```python
from build123d import *

# Parameters (mm, degrees)
F0_R     = 9
F1_DEPTH = 3


with BuildPart() as f1:
    # F0 (on Front) → F1 (new body)
    with BuildSketch(Plane.XZ):
        with BuildLine():
            Line((1.35, 24.837218), (1.35, 13.856218))
            Line((1.35, 13.856218), (-1.35, 13.856218))
            Line((-1.35, 13.856218), (-1.35, 24.837218))
            ThreePointArc((-1.35, 24.837218), (-9.30431, 23.022838), (-16.250873, 18.744019))
            Line((-16.250873, 18.744019), (-8.48636, 10.979053))
            Line((-8.48636, 10.979053), (-10.424493, 9.099692))
            Line((-10.424493, 9.099692), (-18.189233, 16.864432))
            ThreePointArc((-18.189233, 16.864432), (-22.849106, 9.663922), (-24.801066, 1.312179))
            Line((-24.801066, 1.312179), (-13.820066, 1.312179))
            Line((-13.820066, 1.312179), (-13.811545, -1.388101))
            Line((-13.811545, -1.388101), (-24.792545, -1.388101))
            ThreePointArc((-24.792545, -1.388101), (-22.854652, -9.674423), (-18.233002, -16.819974))
            Line((-18.233002, -16.819974), (-10.468263, -9.055235))
            Line((-10.468263, -9.055235), (-8.311446, -11.123312))
            Line((-8.311446, -11.123312), (-16.075972, -18.887838))
            ThreePointArc((-16.075972, -18.887838), (-8.894515, -23.145882), (-0.707747, -24.78329))
            Line((-0.707747, -24.78329), (-0.69587, -13.802296))
            Line((-0.69587, -13.802296), (2.003764, -13.757801))
            Line((2.003764, -13.757801), (1.70544, -24.734748))
            ThreePointArc((1.70544, -24.734748), (9.667631, -22.834323), (16.579394, -18.44848))
            Line((16.579394, -18.44848), (8.911142, -10.588437))
            Line((8.911142, -10.588437), (10.82033, -8.679249))
            Line((10.82033, -8.679249), (18.48873, -16.539148))
            ThreePointArc((18.48873, -16.539148), (22.915536, -9.529923), (24.788649, -1.4542))
            Line((24.788649, -1.4542), (13.807649, -1.4542))
            Line((13.807649, -1.4542), (13.823381, 1.245754))
            Line((13.823381, 1.245754), (24.804381, 1.2458))
            ThreePointArc((24.804381, 1.2458), (22.970893, 9.47684), (18.488676, 16.619769))
            Line((18.488676, 16.619769), (10.723937, 8.85503))
            Line((10.723937, 8.85503), (8.814749, 10.764218))
            Line((8.814749, 10.764218), (16.579488, 18.528958))
            ThreePointArc((16.579488, 18.528958), (9.50343, 22.98359), (1.35, 24.837218))
        make_face()
        Circle(F0_R, mode=Mode.SUBTRACT)
    extrude(amount=F1_DEPTH)


solid = f1.part
```
Read the model definition and answer for the solid it produces. Units are mm, in the model's axes. A direction names the side the tool comes from. Coordinates: 2 decimals unless noted, no trailing zeros. Order: outer loops, then holes, each group sorted by start corner. A loop starts at its lowest first (then second) coordinate and runs counter-clockwise, first axis right, second up. Notation, with made-up numbers: (-29.75, 41.5) - (-3.75, 41.5) arc R25 cw to (-3.75, 66.5) - close; hole circle Ø5 at (34.25, -3). An arc over 180 degrees is marked (long way). Answer as a JSON object with one key per item and string values. Group by question number.
Item 1: Section A-A (x = 12.5) is taken. Give the vertices of the cut face in (y, z), plus the area to 3 significant figures.
Item 2: Section D-D (x = 0) is taken. Give the vertices of the cut face in (y, z), plus the area to 3 significant figures.
Item 3: Section C-C (z = 14.5) is taken. Give the vertices of the cut face in (x, y), plus the area to 3 significant figures.
Item 4: Flat-ended cylindrical pins translate along their axes: P1, Ø1.5, axis at y = -1, z = 18, coming from the +X side; P2, Ø1.5, axis at x = 20, y = -2, coming from the +Z side; P3, Ø0.9, axis at x = 21.5, y = -2, coming from the -Z side; P4, Ø11, axis at x = 0, z = 0, coming from the -Y side. Find the tip coordinate at first contact, or state that the pin passes through.
Item 5: Consider probe 1 along Z at (x, y) = (0, -1.05); probe 2 along Z at (x, y) = (12, -1.3); probe 3 along Z at (x, y) = (11, -2.8). Determine where each line is inside the solid, lowest interval first. Write a range as from..to.
Item 6: The mould has two halves that part along Z. Classify faces 4 (the face through (11, -3, 0)), 5 (the face through (-1.172, -1.479, 8.923)), 6 (the face through (-22.802, -1.479, 9.775)), 7 (the face through (12.64, -1.48, 14.59)): +Z half, -Z half, draft (parallel to the pull), parting line (faces both ways), or undercut.
Item 7: A tool of negligible diameter and unlimited length cuts with its end or side. For faces 1 (the face through (9.78, -1.48, 9.8)), 2 (the face through (9.61, -1.48, 22.94)), 3 (the face through (1.35, -1, 19)), from which of +Z, -Z, +X, -X, +Y, -Y can it reach the whole face along a straight path? Write none if from no direction.
Results are:
{
 "1": {"outline": "(-3, -21.42) - (0, -21.42) - (0, -14.27) - (-3, -14.27) - close; (-3, -10.4) - (0, -10.4) - (0, 10.63) - (-3, 10.63) - close; (-3, 14.45) - (0, 14.45) - (0, 21.5) - (-3, 21.5) - close", "area": "106 mm^2"},
 "2": {"outline": "(-3, -13.79) - (0, -13.79) - (0, -9) - (-3, -9) - close; (-3, 9) - (0, 9) - (0, 13.86) - (-3, 13.86) - close", "area": "28.9 mm^2"},
 "3": {"outline": "(-20.12, -3) - (-15.82, -3) - (-15.82, 0) - (-20.12, 0) - close; (-12.01, -3) - (-1.35, -3) - (-1.35, 0) - (-12.01, 0) - close; (1.35, -3) - (12.55, -3) - (12.55, 0) - (1.35, 0) - close; (16.37, -3) - (20.19, -3) - (20.19, 0) - (16.37, 0) - close", "area": "89.9 mm^2"},
 "4": {"P1": "stops at x = 16.58", "P2": "stops at z = 15.73", "P3": "stops at z = -13.14", "P4": "passes through"},
 "5": {"probe 1": "z = -13.79..-9, 9..13.86", "probe 2": "z = -21.7..-13.75, -9.89..10.13, 13.95..21.78", "probe 3": "z = -22.22..-12.73, -8.86..9.13, 12.95..22.3"},
 "6": {"face 4": "draft", "face 5": "undercut", "face 6": "+Z half", "face 7": "undercut"},
 "7": {"face 1": "+Y, -Y", "face 2": "+Z, +X, +Y, -Y", "face 3": "+Z, +Y, -Y"}
}
